For this review, take the finished solid that the model builds, in its own axes (mm). Face numbers are marked on the shaded views. A direction names the side the tool comes from. Round coordinates to 2 decimals unless told otherwise and drop trailing zeros. Loops run counter-clockwise (first coordinate to the right, second up) from the corner with the lowest first, then second, coordinate; pieces in that order, holes last.
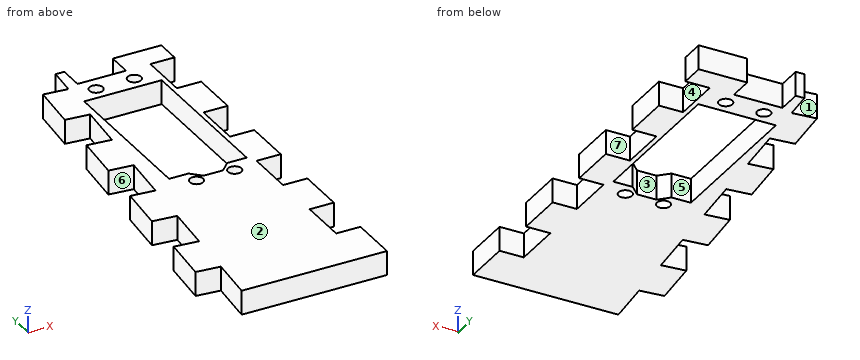
```python
from build123d import *

# Parameters (mm, degrees)
BOSS_EXTRUDE1_DEPTH = 6.35
SKETCH4_R           = 1.75
CUT_EXTRUDE1_DEPTH  = 7.35
SKETCH6_W           = 6.35
SKETCH6_H           = 12.7
CUT_EXTRUDE2_DEPTH  = 7.35
LPATTERN1_COUNT     = 5
LPATTERN1_PITCH     = 25.4
SKETCH7_W           = 12.7
SKETCH7_H           = 6.35
CUT_EXTRUDE3_DEPTH  = 7.35
CUT_EXTRUDE4_DEPTH  = 7.35
LPATTERN2_COUNT     = 5
LPATTERN2_PITCH     = 25.4


with BuildPart() as part:
    # Sketch2 → Boss-Extrude1 (new body)
    with BuildSketch(Plane.XY):
        Polygon((19.565934594, 203.2), (29.960337347, 311.15), (64.008541785, 311.15), (64.008541785, 203.2), align=None)
    extrude(amount=BOSS_EXTRUDE1_DEPTH)

    # Sketch4 → Cut-Extrude1 (cut, through all)
    with BuildSketch(Plane.XY.offset(6.35)):
        with Locations((41.228541785, 300.7)):
            Circle(SKETCH4_R)
        with Locations((51.228541785, 300.7)):
            Circle(SKETCH4_R)
        with Locations((41.228541785, 252.7)):
            Circle(SKETCH4_R)
        with Locations((51.228541785, 252.7)):
            Circle(SKETCH4_R)
        Polygon((56.388541785, 256.38), (56.388541785, 297.02), (36.068541785, 297.02), (36.068541785, 256.38), (41.148541785, 256.38), (43.688541785, 253.84), (48.768541785, 253.84), (51.308541785, 256.38), align=None)
    extrude(amount=-CUT_EXTRUDE1_DEPTH, mode=Mode.SUBTRACT)

    # Sketch6 → Cut-Extrude2 (cut, through all)
    with BuildSketch(Plane.XY.offset(6.35)):
        with Locations((60.833541785, 298.45)):
            Rectangle(SKETCH6_W, SKETCH6_H)
    cut_extrude2 = extrude(amount=-CUT_EXTRUDE2_DEPTH, mode=Mode.SUBTRACT)

    # LPattern1: Cut-Extrude2 ×5
    with Locations(*[(0, -i * LPATTERN1_PITCH, 0) for i in range(1, LPATTERN1_COUNT)]):
        add(cut_extrude2, mode=Mode.SUBTRACT)

    # Sketch7 → Cut-Extrude3 (cut, through all)
    with BuildSketch(Plane.XY.offset(6.35)):
        with Locations((44.958541785, 307.975)):
            Rectangle(SKETCH7_W, SKETCH7_H)
    extrude(amount=-CUT_EXTRUDE3_DEPTH, mode=Mode.SUBTRACT)

    # Sketch8 → Cut-Extrude4 (cut, through all)
    with BuildSketch(Plane.XY.offset(6.35)):
        Polygon((19.565934594, 203.2), (20.783175651, 215.841531719), (27.10394151, 215.232911191), (25.886700453, 202.591379471), align=None)
    cut_extrude4 = extrude(amount=-CUT_EXTRUDE4_DEPTH, mode=Mode.SUBTRACT)

    # LPattern2: Cut-Extrude4 ×5
    with Locations(*[Vector(0.095845753, 0.995396198, 0) * (i * LPATTERN2_PITCH) for i in range(1, LPATTERN2_COUNT)]):
        add(cut_extrude4, mode=Mode.SUBTRACT)


solid = part.part
```
(1) Insertion check: pin 1 Ø12 at (x, y) = (46, 287.5) entering from +Z; pin 2 Ø1.9 at (y, z) = (283, 3) entering from -X; pin 3 Ø2.5 at (x, z) = (46.5, 3.5) entering from +Y. Each pin has a flat end and moves straight along its axis. Give the tip position at first contact, or say it passes through.
(2) Add section A-A (x = 45). Give the boundary of the cut face in (y, z), plus the area to 3 significant figures.
(3) For the marked faces 5, 6 and 7, list the 3-axis set-ups (+Z, -Z, +X, -X, +Y, -Y) from which the entire face can be reached by the end or side of a thin tool; tool diameter is ignored.
(4) Add section C-C (y = 300.7). Give the boundary of the cut face in (x, z), plus the area to 3 significant figures.
(5) The part is to be moulded in two halves that separate along Y. For the marked faces 1, 2, 3 and 4, say which applies: pulls with the +Y half, pulls with the -Y half, needs draft (parallel to the pull), parting line crosses it, or undercut.
(6) Add section D-D (z = 1). Give the number of separate pieces and of enclosed holes in the cut face, plus the area to 3 significant figures.
(7) Add section B-B (y = 274.5). Give the boundary of the cut face in (x, z).
(8) For L1, parallel to Y at x = 44, z = 1.75; L2, parallel to X at y = 299.5, z = 2; L3, parallel to Y at x = 62, z = 4.5, list the stretches that pass through material, from the lowest coordinate up.
Outcome:
1. pin 1: passes through
1. pin 2: stops at x = 33.54
1. pin 3: stops at y = 304.8
2. outline: (203.2, 0) - (253.84, 0) - (253.84, 6.35) - (203.2, 6.35) - close; (297.02, 0) - (304.8, 0) - (304.8, 6.35) - (297.02, 6.35) - close
2. area: 371 mm2
3. face 5: +Z, -Z
3. face 6: +Z, -Z, -X
3. face 7: +Z, -Z, +X
4. outline: (28.95, 0) - (39.48, 0) - (39.48, 6.35) - (28.95, 6.35) - close; (42.98, 0) - (49.48, 0) - (49.48, 6.35) - (42.98, 6.35) - close; (52.98, 0) - (57.66, 0) - (57.66, 6.35) - (52.98, 6.35) - close
4. area: 138 mm2
5. face 1: pulls with the +Y half
5. face 2: needs draft
5. face 3: undercut
5. face 4: undercut
6. separate pieces: 1
6. enclosed holes: 5
6. area: 2,580 mm2
7. outline: (26.43, 0) - (36.07, 0) - (36.07, 6.35) - (26.43, 6.35) - close; (56.39, 0) - (57.66, 0) - (57.66, 6.35) - (56.39, 6.35) - close
8. L1: y = 203.2 to 253.84, 297.02 to 304.8
8. L2: x = 28.84 to 39.95, 42.5 to 49.95, 52.5 to 57.66
8. L3: y = 203.2 to 215.9, 228.6 to 241.3, 254 to 266.7, 279.4 to 292.1, 304.8 to 311.15
